Verification items for the finished model (mm, model axes). A direction names the side the tool comes from. Give positions to 0.01 mm unless a question says otherwise; leave off trailing zeros. Write each loop counter-clockwise with the first axis right and the second up, starting at its lowest first coordinate (ties: lowest second). Pieces come first, ordered by that corner, then holes.
Autodesk Fusion 360 part; units mm, degrees
sketch "Sketch1" plane through (0, 0, 0) normal (0, 0, 1) x (1, 0, 0)
  circle A0 centre (0, 0) radius 4.7625
  dimension "d1" = 9.525
extrude "Extrude1" add sketch "Sketch1" along normal blind 11.43 makes body 1
sketch "Sketch2" plane through (0, 0, 11.43) normal (0, 0, 1) x (1, 0, 0)
  circle A0 centre (0, 0) radius 4.7625
  line L0 (-2.3876, 2.5527) -> (-2.3876, -2.5527)
  line L1 (2.3876, -2.5527) -> (2.3876, 2.5527)
  line L2 (2.3876, 2.5527) -> (-2.3876, -2.5527) construction
  line L3 (-2.3876, 2.5527) -> (2.3876, -2.5527) construction
  arc A1 (2.3876, 2.5527) -> (-2.3876, 2.5527) centre (0, 0.0915) ccw
  arc A2 (-2.3876, -2.5527) -> (2.3876, -2.5527) centre (0, -0.0771) ccw
  dimension "d4" = 5.1054
  dimension "d5" = 4.7752
  dimension "d6" = 3.429
  dimension "d7" = 3.4394
extrude "Extrude2" cut sketch "Sketch2" against normal blind 5.1562 contours L0 L1 A1 A2 bodies 1
extrude "Extrude3" cut 1 faces at (0.58, -0.1002, 0) along direction (0, 0, 1) blind 3.048 on bodies 1 bodies 1
sketch "Sketch3" plane through (0, 0, 3.048) normal (0, 0, -1) x (-1, 0, 0)
  circle A0 centre (0, 0) radius 4.7625
  line L0 (-10.795, 5.334) -> (10.795, 5.334)
  line L1 (10.795, 5.334) -> (10.795, -5.334)
  line L2 (10.795, -5.334) -> (-10.795, -5.334)
  line L3 (-10.795, -5.334) -> (-10.795, 5.334)
  line L4 (-10.795, 5.334) -> (10.795, -5.334) construction
  line L5 (10.795, 5.334) -> (-10.795, -5.334) construction
  dimension "d12" = 21.59
  dimension "d13" = 10.668
extrude "Extrude5" add sketch "Sketch3" against normal blind 2.54 bodies 1
extrude "Extrude4" add sketch "Sketch3" along normal blind 2.54 contours A0 | L0 L1 L2 L3 bodies 1
sketch "Sketch4" plane through (0, 0, 0.508) normal (0, 0, -1) x (-1, 0, 0)
  line L0 (-10.795, -5.334) -> (10.795, -5.334)
  line L1 (10.795, -5.334) -> (10.795, 5.334)
  line L2 (10.795, 5.334) -> (-10.795, 5.334)
  line L3 (-10.795, 5.334) -> (-10.795, -5.334)
  circle A0 centre (0, 0) radius 1.5
  circle A1 centre (-7.62, 0) radius 1.5
  circle A2 centre (7.62, 0) radius 1.5
  dimension "d18" = 3
  dimension "d19" = 3
  dimension "d20" = 3
extrude "Extrude6" cut sketch "Sketch4" against normal blind 13.97 contours A0 | A1 | A2 bodies 1
sketch "Sketch5" plane through (0, 0, 0.508) normal (0, 0, -1) x (-1, 0, 0)
  circle A0 centre (-7.62, 0) radius 1.5
  circle A1 centre (0, 0) radius 1.5
  circle A2 centre (7.62, 0) radius 1.5
  line L0 (-10.795, -5.334) -> (10.795, -5.334)
  line L1 (10.795, -5.334) -> (10.795, 5.334)
  line L2 (10.795, 5.334) -> (-10.795, 5.334)
  line L3 (-10.795, 5.334) -> (-10.795, -5.334)
  line L4 (-2.3876, -2.5527) -> (-2.3876, 2.5527)
  line L5 (-2.3876, 2.5527) -> (-2.3876, -2.5527)
  line L6 (2.3876, 2.5527) -> (2.3876, -2.5527)
  arc A3 (2.3876, 2.5527) -> (-2.3876, 2.5527) centre (0, 0.0915) ccw
  arc A4 (-2.3876, -2.5527) -> (2.3876, -2.5527) centre (0, -0.0771) ccw
extrude "Extrude7" add sketch "Sketch5" along normal blind 4.191 contours L4 L5 L6 A3 A4 bodies 1
fillet "Fillet1" radius 0.508 13 edges at (-10.795, -5.334, 3.048) (-10.795, 5.334, 3.048) (10.795, 5.334, 3.048) (10.795, -5.334, 3.048) (10.795, 0, 5.588) (10.795, 0, 0.508) (0, 5.334, 0.508) (0, 5.334, 5.588) (-10.795, 0, 5.588) (-10.795, 0, 0.508) (0, -5.334, 5.588) (0, -5.334, 0.508) (-4.4402, -1.7222, 11.43) on bodies 1
sketch "Sketch6" plane through (0, 0, 0.508) normal (0, 0, -1) x (-1, 0, 0)
  circle A0 centre (7.62, 0) radius 1.5
  circle A1 centre (-7.62, 0) radius 1.5
  line L0 (2.3876, 2.5527) -> (2.3876, -2.5527)
  arc A2 (-2.3876, -2.5527) -> (2.3876, -2.5527) centre (0, -0.0771) ccw
  line L1 (-2.3876, -2.5527) -> (-2.3876, 2.5527)
  arc A3 (2.3876, 2.5527) -> (-2.3876, 2.5527) centre (0, 0.0915) ccw
  line L2 (10.287, -4.826) -> (10.287, 4.826)
  line L3 (10.287, 4.826) -> (-10.287, 4.826)
  line L4 (-10.287, 4.826) -> (-10.287, -4.826)
  line L5 (-10.287, -4.826) -> (10.287, -4.826)
  circle A4 centre (0, 0.0915) radius 17.2202
  circle A5 centre (-7.62, 0) radius 1.5
  line L6 (-2.3876, 2.5527) -> (-2.3876, -2.5527)
  arc A6 (2.3876, 2.5527) -> (-2.3876, 2.5527) centre (0, 0.0915) ccw
  line L7 (2.3876, -2.5527) -> (2.3876, 2.5527)
  arc A7 (-2.3876, -2.5527) -> (2.3876, -2.5527) centre (0, -0.0771) ccw
  circle A8 centre (7.62, 0) radius 1.5
extrude "Extrude8" add sketch "Sketch6" along normal blind 3.81 separate body contours L2 L3 L4 L5 | A4 makes body 2
hidden bodies 2
Item 1: Release check for a two-part mould opening along X. For faces 5 (the face through (0, -5.334, 3)), 6 (the face through (-0.037, -3.516, -1.558)), 7 (the face through (1.5, -0.07, 1.37)) record: released by +X, released by -X, zero draft, split by the parting line, or undercut.
Answer key:
face 5: zero draft
face 6: split by the parting line
face 7: undercut
Item 2: Scan lines: line 1 along Y through (x, z) = (0, 1); line 2 along Z through (x, y) = (7.5, -2.75); line 3 along Z through (x, y) = (2, 3). Record each from-to range of solid material in increasing order.
Answer key:
line 1: y = -5.33 to -1.5, 1.5 to 5.33
line 2: z = 0.51 to 5.59
line 3: z = 0.51 to 11.43
Item 3: Set-up check for faces 1 (the face through (-0.037, -3.516, 8.888)), 2 (the face through (2.388, 0, -2)), 3 (the face through (-2.388, 0, -2)), 4 (the face through (0.04, 3.52, -1.56)): record each of +Z, -Z, +X, -X, +Y, -Y from which the full face is reachable in a straight line by a thin tool's end or side.
Answer key:
face 1: +Z
face 2: -Z, +X, +Y, -Y
face 3: -Z, -X, +Y, -Y
face 4: -Z, +Y
Item 4: Sectioned sample at C-C on y = 0. State how many separate pieces and enclosed holes the cut face has, then the cut area to 3 significant figures.
Answer key:
separate pieces: 4
enclosed holes: 0
area: 100 mm2
Item 5: Sectioned sample at D-D on z = -2. Record the cut outline in (x, y).
Answer key:
outline: (-2.39, -2.55) arc R3.44 ccw to (2.39, -2.55) - (2.39, 2.55) arc R3.43 ccw to (-2.39, 2.55) - close; hole circle Ø3 at (0, 0)
Item 6: Sectioned sample at A-A on x = 7.62. Record the cut outline in (y, z).
Answer key:
outline: (-5.33, 1.02) arc R0.51 ccw to (-4.83, 0.51) - (-1.5, 0.51) - (-1.5, 5.59) - (-4.83, 5.59) arc R0.51 ccw to (-5.33, 5.08) - close; (1.5, 0.51) - (4.83, 0.51) arc R0.51 ccw to (5.33, 1.02) - (5.33, 5.08) arc R0.51 ccw to (4.83, 5.59) - (1.5, 5.59) - close
Item 7: Depth check by flat-ended pin: pin 1 (1 mm diameter, centred on x = 7.5, y = -2.5, fed in from +Z); pin 2 (3.5 mm diameter, centred on x = 7.62, y = 0, fed in from -Z); pin 3 (4 mm diameter, centred on y = -0.5, z = 9, fed in from -X). Enter the tip coordinate at first touch or a pass-through.
Answer key:
pin 1: stops at z = 5.59
pin 2: stops at z = 0.51
pin 3: stops at x = -4.76
Item 8: Sectioned sample at B-B on z = 4.5. Record the cut outline in (x, y) (3 decimals).
Answer key:
outline: (-10.795, -4.826) arc R0.508 ccw to (-10.287, -5.334) - (10.287, -5.334) arc R0.508 ccw to (10.795, -4.826) - (10.795, 4.826) arc R0.508 ccw to (10.287, 5.334) - (-10.287, 5.334) arc R0.508 ccw to (-10.795, 4.826) - close; hole circle Ø3 at (-7.62, 0); hole circle Ø3 at (0, 0); hole circle Ø3 at (7.62, 0)
